Answer from the drawing. Dimensions are ordinates in mm from the lowest x, y and z of the part. A direction names the side the tool comes from. Give positions to 0.01 mm unless a question says otherwise; leave off trailing zeros. Write each loop counter-clockwise with the first axis right and the second up, starting at its lowest first coordinate (ties: lowest second). Pieces come first, ordered by that corner, then holes. Notation, with made-up numbers: (85.5, 70.5) -> (130.5, 70.5) arc R18 cw to (130.5, 83.5) -> close; hole circle Ø5 at (4.5, 23). An arc over 180 degrees is marked (long way). Use a Markdown table: item, result. Add a question column.
Q1. Each of these flat-tipped pins is pushed along its axis until it touches: pin 1 Ø16 at (x, z) = (40, 15) entering from -Y; pin 2 Ø18 at (x, y) = (57.5, 22) entering from +Z. Where does it stop, or does it pass through?
Q2. Section A-A, the plane z = 15 is taken. Give the vertices of the cut face in (x, y).
Q3. Section C-C, the plane y = 38 is taken. Give the vertices of the cut face in (x, z).
Q4. Section D-D, the plane z = 68 is taken. Give the vertices of the cut face in (x, y).
Q5. For the marked faces 1 and 2, determine the directions among +Z, -Z, +X, -X, +Y, -Y from which every point of the face is accessible in a straight line to the end or side of a thin tool.
Q6. Consider line 1 (Z direction, x = 40, y = 6); line 2 (Z direction, x = 44, y = 18.5); line 3 (Y direction, x = 45, z = 9). Determine where each line is inside the solid, lowest interval first.
Q7. Section B-B, the plane x = 10 is taken. Give the vertices of the cut face in (y, z).
Q8. For a pull along X with two mould halves and no side action, classify the marked faces 3, 4, 5 and 6 as pulls with the +X half, pulls with the -X half, needs draft (parallel to the pull), parting line crosses it, or undercut.
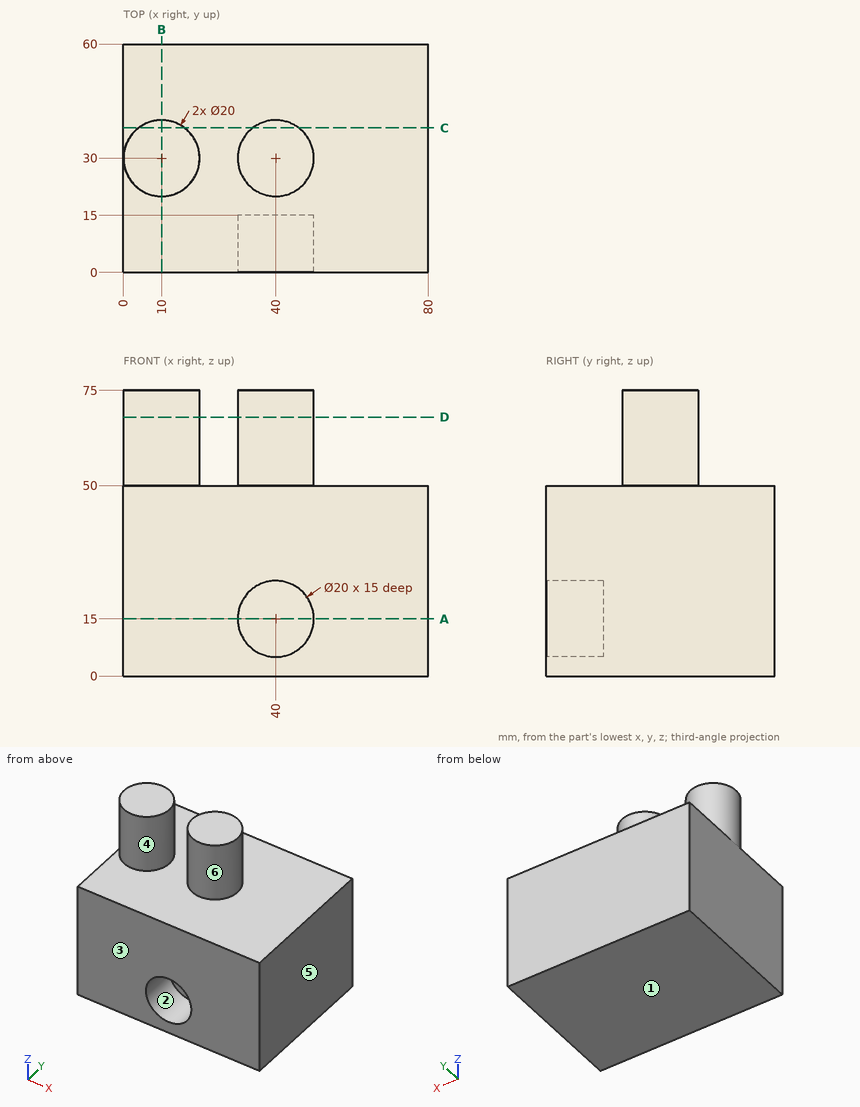
Result set:
| question | item | result |
|---|---|---|
| 1 | pin 1 | stops at y = 15 |
| 1 | pin 2 | stops at z = 50 |
| 2 | outline | (0, 0) -> (30, 0) -> (30, 15) -> (50, 15) -> (50, 0) -> (80, 0) -> (80, 60) -> (0, 60) -> close |
| 3 | outline | (0, 0) -> (80, 0) -> (80, 50) -> (46, 50) -> (46, 75) -> (34, 75) -> (34, 50) -> (16, 50) -> (16, 75) -> (4, 75) -> (4, 50) -> (0, 50) -> close |
| 4 | outline | circle Ø20 at (10, 30); circle Ø20 at (40, 30) |
| 5 | face 1 | -Z, +X, -X, +Y, -Y |
| 5 | face 2 | -Y |
| 6 | line 1 | z = 0 to 5, 25 to 50 |
| 6 | line 2 | z = 0 to 50 |
| 6 | line 3 | y = 15 to 60 |
| 7 | outline | (0, 0) -> (60, 0) -> (60, 50) -> (40, 50) -> (40, 75) -> (20, 75) -> (20, 50) -> (0, 50) -> close |
| 8 | face 3 | needs draft |
| 8 | face 4 | undercut |
| 8 | face 5 | pulls with the +X half |
| 8 | face 6 | undercut |
